Model file for the job. Use its own axes, mm. A direction names the side the tool comes from. Coordinates: 2 decimals unless noted, no trailing zeros. Write item = value, one per line. Start each with the question number.
from build123d import *

# Parameters (mm, degrees)
BOSS_EXTRUDE1_DEPTH = 3.175
CUT_EXTRUDE1_DEPTH  = 7.3500001
FILLET1_R           = 2.54
CUT_EXTRUDE2_DEPTH  = 7.62


with BuildPart() as part:
    # Sketch1 → Boss-Extrude1 (new body, symmetric)
    with BuildSketch(Plane.XY):
        with BuildLine():
            Line((499.61002795, -53.470702797), (1046.28548189, -53.470702797))
            add(Edge.make_bspline(
                [(2669.54, -9.569049356), (2615.393603553, -13.17073937), (2561.080658619, -16.536108081), (2506.205230446, -19.758621957), (2430.209106802, -23.505211705), (2354.212983157, -26.631486423), (2332.570330468, -27.480988169), (2156.268639429, -34.377768543), (1979.966947376, -41.628631248), (1824.114277635, -52.771265877), (1636.928606778, -53.579569849), (1449.742935921, -53.454024613), (1418.006730935, -53.470702797), (1324.899336146, -53.470702797), (1231.791940344, -53.470702797), (1170.441269319, -53.470702797), (1108.784075813, -53.470702797), (1047.126882346, -53.470702797), (1046.846414188, -53.470702797), (1046.565947184, -53.470702797), (1046.28548189, -53.470702797)],
                knots=[103.698913506, 103.698913506, 103.698913506, 103.698913506, 103.698913506, 103.698913506, 130.927896619, 130.927896619, 130.927896619, 141.337054719, 141.337054719, 141.337054719, 218.101815019, 218.101815019, 218.101815019, 233.772059419, 233.772059419, 233.772059419, 264.077723219, 264.077723219, 264.077723219, 264.2162088, 264.2162088, 264.2162088, 264.2162088, 264.2162088, 264.2162088], degree=5))
            Line((2669.54, -9.569049356), (2669.54, 9.5231025))
            add(Edge.make_bspline(
                [(2669.54, 9.5231025), (2667.126494524, 9.36235515), (2659.861586685, 8.880281494), (2635.666282302, 7.292469146), (2596.857665529, 4.826056853), (2545.729743039, 1.758344093), (2494.405305707, -1.098555235), (2451.533022267, -3.266573297), (2417.198316756, -4.86708361), (2391.457076919, -6.003589235), (2365.634736307, -7.086854581), (2339.546284672, -8.137729944), (2313.466132974, -9.165138371), (2287.612375486, -10.179478215), (2261.763347437, -11.201032297), (2227.285329715, -12.583842557), (2184.175569393, -14.36607236), (2132.429066114, -16.607427868), (2063.4255234, -19.708920485), (1977.174907635, -23.700543313), (1873.732451432, -28.149389221), (1770.37461881, -31.657468649), (1667.085687813, -33.793117556), (1581.011094491, -34.383188831), (1512.07397126, -34.4278026), (1443.061513477, -34.409510402), (1356.800927879, -34.424432812), (1218.794626954, -34.418464788), (1115.289022786, -34.420702797), (1046.28548189, -34.420702797)],
                knots=[103.571582669, 103.571582669, 103.571582669, 103.571582669, 104.300777207, 105.766098403, 110.877392287, 115.98868617, 121.099980054, 126.211273938, 128.76692088, 131.322567822, 133.878214764, 136.433861706, 138.989508647, 141.545155589, 144.100802531, 146.656449473, 151.767743357, 156.879037241, 161.990331124, 172.212918892, 182.43550666, 192.658094427, 202.880682195, 213.103269962, 218.214563846, 223.32585773, 233.548445497, 243.771033265, 264.2162088, 264.2162088, 264.2162088, 264.2162088], degree=3))
            Line((1046.28548189, -34.420702797), (499.61002795, -34.420702797))
            add(Edge.make_bspline(
                [(499.61002795, -34.420702797), (488.614737518, -34.420702797), (472.236395365, -34.420702798), (449.940231846, -34.420702794), (427.771305695, -34.42070281), (405.874681663, -34.420702712), (384.584909128, -34.420702942), (368.900229326, -34.420702244), (353.376568613, -34.420704862), (332.608466435, -34.420689186), (306.287754853, -34.420570006), (274.023487704, -34.420538256), (252.271015965, -34.420709741), (241.425150134, -34.420702761)],
                knots=[19.90682951, 19.90682951, 19.90682951, 19.90682951, 23.220120017, 24.876765271, 26.533410525, 29.846701033, 31.503346286, 33.15999154, 34.816636794, 36.473282048, 39.786572556, 43.099863063, 46.413153571, 46.413153571, 46.413153571, 46.413153571], degree=3))
            add(Edge.make_bspline(
                [(241.425150134, -34.420702761), (239.394928853, -34.420701455), (235.322322927, -34.420495867), (227.274423443, -34.398702533), (217.319360062, -34.297466855), (205.530690077, -33.976385563), (189.963341914, -33.212641271), (170.696984653, -31.543495194), (147.533261232, -28.314398128), (125.482753206, -24.202109872), (109.358914834, -20.622537553), (100.964116069, -18.612521054), (99.06, -18.149327722)],
                knots=[0, 0, 0, 0, 0.622088422, 1.244176844, 2.488353689, 3.732530533, 4.976707377, 7.465061066, 9.953414755, 12.441768444, 14.55823542, 15.180323842, 15.180323842, 15.180323842, 15.180323842], degree=3))
            Line((99.06, -18.149327722), (99.06, -37.741485304))
            add(Edge.make_bspline(
                [(241.425137875, -53.470702761), (224.286916993, -53.470691732), (207.149474967, -53.467315374), (190.203897513, -52.686577078), (161.734965878, -49.987457476), (133.266034188, -45.175583375), (121.749620566, -42.910592695), (110.349390726, -40.420274627), (99.06, -37.741485304)],
                knots=[0, 0, 0, 0, 0, 0, 8.71381608, 8.71381608, 8.71381608, 14.701907176, 14.701907176, 14.701907176, 14.701907176, 14.701907176, 14.701907176], degree=5))
            add(Edge.make_bspline(
                [(499.61002795, -53.470702797), (492.136820835, -53.470702797), (484.754348064, -53.470702797), (477.443025859, -53.470702797), (448.516583145, -53.470702797), (419.590140517, -53.470702797), (398.368118521, -53.470702797), (355.647540186, -53.470702797), (312.926961851, -53.470702797), (289.235090436, -53.470293029), (265.364963651, -53.470705034), (241.4948369, -53.470702789), (241.471603891, -53.470702785), (241.448370882, -53.470702776), (241.425137875, -53.470702761)],
                knots=[19.90682951, 19.90682951, 19.90682951, 19.90682951, 19.90682951, 19.90682951, 23.637897311, 23.637897311, 23.637897311, 34.276545571, 34.276545571, 34.276545571, 46.401340901, 46.401340901, 46.401340901, 46.413153571, 46.413153571, 46.413153571, 46.413153571, 46.413153571, 46.413153571], degree=5))
        make_face()
    extrude(amount=BOSS_EXTRUDE1_DEPTH, both=True)

    # Sketch2 → Cut-Extrude1 (cut, through all)
    with BuildSketch(Plane.XY.offset(3.175)):
        with BuildLine():
            add(Edge.make_bspline(
                [(2312.9875, -9.183260037), (2304.505441691, -9.516700376), (2287.441020622, -10.186250162), (2261.763347437, -11.201032297), (2228.230552004, -12.545932515), (2203.310445107, -13.575047161), (2187.00995947, -14.263260037)],
                knots=[139.04033329, 139.04033329, 139.04033329, 139.04033329, 141.545155589, 144.100802531, 146.656449473, 151.487488909, 151.487488909, 151.487488909, 151.487488909], degree=3))
            Line((2187.00995947, -14.263260037), (2312.9875, -14.263260037))
            Line((2312.9875, -14.263260037), (2312.9875, -9.183260037))
        make_face()
    extrude(amount=-CUT_EXTRUDE1_DEPTH, mode=Mode.SUBTRACT)

    # Fillet1
    fillet1_edges = [part.edges().sort_by_distance(p)[0] for p in [
        (2669.54, -9.569049356, -1.5875),
        (2669.54, 9.5231025, -1.5875),
        (99.06, -37.741485304, -1.5875),
        (99.06, -18.149327722, -1.5875),
        (2312.9875, -9.183260037, 1.5875),
        (2312.9875, -14.263260037, 0),
    ]]
    fillet(fillet1_edges, radius=FILLET1_R)

    # Sketch3 → Cut-Extrude2 (cut)
    with BuildSketch(Plane.XY.offset(3.175)):
        Polygon((821.518882755, -34.420702797), (819.047328197, -41.874419167), (833.004793216, -46.384200616), (830.756310042, -53.470702797), (833.004793216, -88.377214401), (71.333278148, -146.659078969), (65.822633249, 75.523734032), (821.518882755, 94.266739515), align=None)
        Polygon((1181.433983433, -34.420040525), (1177.136382458, -39.41105826), (1185.135968065, -43.161373269), (1178.857838528, -48.879066642), (1185.135968065, -53.470702797), (1178.857838528, -73.832795228), (2840.460279362, -301.9320282), (2840.460279362, 201.131978716), (1181.433983433, 94.266739515), align=None)
    extrude(amount=-CUT_EXTRUDE2_DEPTH, mode=Mode.SUBTRACT)


solid = part.part
Item 1: Pull direction Y, two halves, no side cores. Call faces 1 (the flat face through (1181.08, -41.26, 0.04)), 2 (the flat face through (1000, -44, 3.175)), 3 (the flat face through (935, -34.421, 0)), 4 (the flat face through (1181.95, -51.14, 0.04)): +Y half, -Y half, draft (parallel to the pull), parting line (faces both ways), or undercut.
Item 2: Probe L1, parallel to X at y = -48.75, z = 2.75; L2, parallel to X at y = -51.25, z = -2.25. List the from-to ranges inside material, lowest first.
Item 3: 3-axis set-ups, long thin cutter, end or side, ignore diameter. For faces 5 (the flat face through (1182.04, -45.98, 0.04)), 6 (the flat face through (831.896, -49.878, 0.044)), 7 (the flat face through (937, -53.471, 0)): which of +Z, -Z, +X, -X, +Y, -Y reach the whole face in a straight line?
Reported:
q1.face_1 = undercut
q1.face_2 = draft
q1.face_3 = +Y half
q1.face_4 = undercut
q2.L1 = 832.25 to 1179
q2.L2 = 831.46 to 1182.1
q3.face_5 = +Z, -Z, +X
q3.face_6 = +Z, -Z, -X
q3.face_7 = +Z, -Z, +X, -X, -Y
